from build123d import *

# Parameters (mm, degrees)
F2_R     = 2.3876
F3_DEPTH = 19.0764
F4_SIZE  = 1.6002
F5_R     = 1.6002
F6_R     = 6.35
F7_DEPTH = 11.1262


with BuildPart() as f1:
    # F0 (on Front) → F1 (revolve)
    with BuildSketch(Plane.XZ):
        Polygon((-19.0627, 3.9751), (-19.0627, 0), (0, 0), (0, 3.9751), (-7.9502, 6.858), (-7.9502, 23.876), (0, 26.67), (0, 36.576), (-19.0754, 36.576), (-19.0754, 26.67), (-11.1252, 23.876), (-11.1252, 6.858), align=None)
    revolve(axis=Axis((-9.53135, 0, 0), (1, 0, 0)))

    # F2 (on face) → F3 (cut, through all)
    with BuildSketch(Plane.YZ):
        Circle(F2_R)
    extrude(amount=-F3_DEPTH, mode=Mode.SUBTRACT)

    # F4
    f4_edges = [f1.edges().sort_by_distance(p)[0] for p in [
        (0, 0, -36.576),
        (-19.0754, 0, -36.576),
    ]]
    chamfer(f4_edges, length=F4_SIZE)

    # F5
    f5_edges = [f1.edges().sort_by_distance(p)[0] for p in [
        (-7.9502, 0, -23.876),
        (-11.1252, 0, -23.876),
        (-7.9502, 0, -6.858),
        (-11.1252, 0, -6.858),
    ]]
    fillet(f5_edges, radius=F5_R)

    # F6 (on face) → F7 (cut, through all)
    with BuildSketch(Plane.YZ.offset(-7.9502)):
        with Locations((0, 15.361061)):
            Circle(F6_R)
        with Locations((-13.303069, 7.680531)):
            Circle(F6_R)
        with Locations((-13.303069, -7.680531)):
            Circle(F6_R)
        with Locations((0, -15.361061)):
            Circle(F6_R)
        with Locations((13.303069, -7.680531)):
            Circle(F6_R)
        with Locations((13.303069, 7.680531)):
            Circle(F6_R)
    extrude(amount=-F7_DEPTH, mode=Mode.SUBTRACT)


solid = f1.part
Model file for the job. Use its own axes, mm. A direction names the side the tool comes from. Give positions to 0.01 mm unless a question says otherwise; leave off trailing zeros. Order: outer loops, then holes, each group sorted by start corner. A loop starts at its lowest first (then second) coordinate and runs counter-clockwise, first axis right, second up. Notation, with made-up numbers: (52, -26) -> (106, -26) arc R21 cw to (106, 4) -> close; hole circle Ø2 at (-9, -7.5). An arc over 180 degrees is marked (long way). Use CSV: the item, a comma, the result in double quotes.
1. Drill centre lines: line 1 along Z through (x, y) = (-9.4, 0); line 2 along Z through (x, y) = (-8, -12); line 3 along Y through (x, z) = (-14.25, 1.5). Where is each one in solid material? Low to high. Write a range as from..to.
Outcome:
line 1,"-36.58..-21.71, -9.01..-2.39, 2.39..9.01, 21.71..36.58"
line 2,"-34.55..-13.9, -1.47..1.47, 13.9..34.55"
line 3,"-36.55..-24.93, -5.52..-1.86, 1.86..5.52, 24.93..36.55"
2. Mould opens along Z. For faces 1 (the cylindrical face through (-9.515, -1.377, 9.162)), 2 (the flat face through (0, 26, 8)) say: +Z half, -Z half, draft (parallel to the pull), parting line (faces both ways), or undercut.
Outcome:
face 1,"undercut"
face 2,"draft"
3. 3-axis set-ups, long thin cutter, end or side, ignore diameter. For faces 3 (the flat face through (-7.95, 10, 0)), 4 (the cylindrical face through (-9.515, 6.057, -13.454)), 5 (the flat face through (-11.125, 10, 0)): which of +Z, -Z, +X, -X, +Y, -Y reach the whole face in a straight line?
Outcome:
face 3,"+X"
face 4,"+X, -X"
face 5,"-X"
4. Drop flat-ended pins along their axis: pin 1 (4.5 mm diameter, centred on y = 0, z = 0, fed in from +X); pin 2 (16.5 mm diameter, centred on y = -13.3, z = -7.68, fed in from +X); pin 3 (1 mm diameter, centred on y = -23, z = -29, fed in from +X); pin 4 (12 mm diameter, centred on y = -15, z = -10, fed in from -X). Give the stop position or say it passes through.
Outcome:
pin 1,"through"
pin 2,"x = -7.69"
pin 3,"x = -1.54"
pin 4,"x = -11.77"
5. Band-saw the part on A-A, the plane y = 0. Count the separate pieces of the cut face and the enclosed holes in it, then the cut area to 3 significant figures.
Outcome:
separate pieces,"4"
enclosed holes,"0"
area,"589 mm²"
6. Band-saw the part on B-B, the plane x = -16.25. Give the cut face in (y, z), then the cut area to 3 significant figures.
Outcome:
outline,"circle Ø73.15 at (0, 0); circle Ø9.99 at (0, 0); hole circle Ø51.35 at (0, 0); hole circle Ø4.78 at (0, 0)"
area,"2,190 mm²"
